from build123d import *

# Parameters (mm, degrees)
F0_R     = 17.85
F1_DEPTH = 1.2
F2_R     = 11.5
F3_DEPTH = 6
F4_W     = 9.2
F4_H     = 18.8
F5_DEPTH = 7.201
F7_DEPTH = 6.7
F8_W     = 11
F8_H     = 25
F9_DEPTH = 4


with BuildPart() as f1:
    # F0 (on Top) → F1 (new body)
    with BuildSketch(Plane.XY):
        Circle(F0_R)
    extrude(amount=F1_DEPTH)

    # F2 (on face) → F3 (join)
    with BuildSketch(Plane.XY.offset(1.2)):
        Circle(F2_R)
    extrude(amount=F3_DEPTH)

    # F4 (on face) → F5 (cut, through all)
    with BuildSketch(Plane.XY.offset(7.2)):
        Rectangle(F4_W, F4_H)
    extrude(amount=-F5_DEPTH, mode=Mode.SUBTRACT)

    # F6 (on face) → F7 (cut)
    with BuildSketch(Plane.XY.offset(7.2)):
        with BuildLine():
            Line((5.4, 10.4), (-5.4, 10.4))
            Line((-5.4, 10.4), (-5.4, 7.4))
            ThreePointArc((-5.4, 7.4), (-5, 7), (-5.4, 6.6))
            Line((-5.4, 6.6), (-5.4, -6.6))
            ThreePointArc((-5.4, -6.6), (-5, -7), (-5.4, -7.4))
            Line((-5.4, -7.4), (-5.4, -10.4))
            Line((-5.4, -10.4), (5.4, -10.4))
            Line((5.4, -10.4), (5.4, -7.4))
            ThreePointArc((5.4, -7.4), (5, -7), (5.4, -6.6))
            Line((5.4, -6.6), (5.4, 6.6))
            ThreePointArc((5.4, 6.6), (5, 7), (5.4, 7.4))
            Line((5.4, 7.4), (5.4, 10.4))
        make_face()
    extrude(amount=-F7_DEPTH, mode=Mode.SUBTRACT)

    # F8 (on face) → F9 (cut)
    with BuildSketch(Plane.XY.offset(7.2)):
        Rectangle(F8_W, F8_H)
    extrude(amount=-F9_DEPTH, mode=Mode.SUBTRACT)


solid = f1.part
Input: part model. Units: mm. Frame: model coordinates. A direction names the side the tool comes from. Coordinates: 2 decimals unless noted, no trailing zeros. Loops run counter-clockwise (first coordinate to the right, second up) from the corner with the lowest first, then second, coordinate; pieces in that order, holes last. Notation, with made-up numbers: (-3, 27.25) -> (21, 27.25) arc R17 cw to (21, 59.25) -> close; hole circle Ø10 at (73.25, 67). An arc over 180 degrees is marked (long way). One line per item, written item: value.
(1) Set-up query: faces 4 (the face through (-0.1, -11.5, 2.2)), 5 (the face through (-5.5, 0, 5)), 6 (the face through (8, 0, 0)), 7 (the face through (-5, 7, 2)). Return all of +Z, -Z, +X, -X, +Y, -Y with unobstructed straight access to the full face (end or side cutting, diameter ignored); none if empty.
Answer below:
face 4: +Z, -Y
face 5: +Z, +Y, -Y
face 6: -Z, +X, -X, +Y, -Y
face 7: +Z
(2) Ray query, line 1 along Y through (x, z) = (4, 0.75); line 2 along X through (y, z) = (4.5, 6.5); line 3 along X through (y, z) = (3, 4.5). Return the intervals inside material, ascending.
Answer below:
line 1: y = -17.4 to -10.4, 10.4 to 17.4
line 2: x = -10.58 to -5.5, 5.5 to 10.58
line 3: x = -11.1 to -5.5, 5.5 to 11.1
(3) Cut plane A-A (y = 0). Output: boundary loops of the cut face in (x, z), then the cut area to 3 significant figures.
Answer below:
outline: (-17.85, 0) -> (-4.6, 0) -> (-4.6, 0.5) -> (-5.4, 0.5) -> (-5.4, 3.2) -> (-5.5, 3.2) -> (-5.5, 7.2) -> (-11.5, 7.2) -> (-11.5, 1.2) -> (-17.85, 1.2) -> close; (4.6, 0) -> (17.85, 0) -> (17.85, 1.2) -> (11.5, 1.2) -> (11.5, 7.2) -> (5.5, 7.2) -> (5.5, 3.2) -> (5.4, 3.2) -> (5.4, 0.5) -> (4.6, 0.5) -> close
area: 103 mm2
(4) Cut plane D-D (z = 4.75). Output: boundary loops of the cut face in (x, y).
Answer below:
outline: (-5.5, -10.1) -> (-5.5, 10.1) arc R11.5 ccw to start; (5.5, -10.1) arc R11.5 ccw to (5.5, 10.1) -> close
(5) Cut plane C-C (x = 0). Output: boundary loops of the cut face in (y, z).
Answer below:
outline: (-17.85, 0) -> (-9.4, 0) -> (-9.4, 0.5) -> (-10.4, 0.5) -> (-10.4, 3.2) -> (-11.5, 3.2) -> (-11.5, 1.2) -> (-17.85, 1.2) -> close; (9.4, 0) -> (17.85, 0) -> (17.85, 1.2) -> (11.5, 1.2) -> (11.5, 3.2) -> (10.4, 3.2) -> (10.4, 0.5) -> (9.4, 0.5) -> close
(6) Cut plane B-B (z = 2). Output: boundary loops of the cut face in (x, y), then the cut area to 3 significant figures.
Answer below:
outline: (-5.4, -10.15) -> (-5.4, -7.4) arc R0.4 ccw to (-5.4, -6.6) -> (-5.4, 6.6) arc R0.4 ccw to (-5.4, 7.4) -> (-5.4, 10.15) arc R11.5 ccw to start; (-4.91, -10.4) arc R11.5 ccw to (4.91, -10.4) -> close; (-4.91, 10.4) -> (4.91, 10.4) arc R11.5 ccw to start; (5.4, -10.15) arc R11.5 ccw to (5.4, 10.15) -> (5.4, 7.4) arc R0.4 ccw to (5.4, 6.6) -> (5.4, -6.6) arc R0.4 ccw to (5.4, -7.4) -> close
area: 192 mm2
(7) Draft query along X for faces 1 (the face through (5.5, 0, 5)), 2 (the face through (11.5, -0.2, 4.2)), 3 (the face through (-11.5, 0.2, 4.2)). Return one class per face: pulls with the +X half, pulls with the -X half, needs draft (parallel to the pull), parting line crosses it, or undercut.
Answer below:
face 1: undercut
face 2: pulls with the +X half
face 3: pulls with the -X half
(8) Pin query (flat end, axial travel): pin 1 Ø1.4 at (y, z) = (9.5, 1.5) entering from -X; pin 2 Ø3 at (y, z) = (-3.5, 5.5) entering from +X; pin 3 Ø1.5 at (y, z) = (-1.5, 2) entering from -X; pin 4 Ø1 at (x, z) = (1.5, 4) entering from +Y. Return the tip coordinate at first contact, or that it passes through.
Answer below:
pin 1: stops at x = -15.49
pin 2: stops at x = 11.32
pin 3: stops at x = -11.48
pin 4: passes through
